```python
from build123d import *

# Parameters (mm, degrees)
F0_R      = 2.75
F1_DEPTH  = 4
F2_R      = 2.75
F3_DEPTH  = 9
F5_DEPTH  = 4
F7_R      = 5.125
F8_DEPTH  = 18.001
F10_DEPTH = 2


with BuildPart() as f1:
    # F0 (on Top) → F1 (new body)
    with BuildSketch(Plane.XY):
        with BuildLine():
            ThreePointArc((85, 25), (82.071068, 32.071068), (75, 35))
            Line((75, 35), (-75, 35))
            ThreePointArc((-75, 35), (-82.071068, 32.071068), (-85, 25))
            Line((-85, 25), (-85, -25))
            ThreePointArc((-85, -25), (-82.071068, -32.071068), (-75, -35))
            Line((-75, -35), (75, -35))
            ThreePointArc((75, -35), (82.071068, -32.071068), (85, -25))
            Line((85, -25), (85, 25))
        make_face()
        with Locations((-74, -25)):
            Circle(F0_R, mode=Mode.SUBTRACT)
        with Locations((74, -25)):
            Circle(F0_R, mode=Mode.SUBTRACT)
        with BuildLine():
            ThreePointArc((61.773717, 13.674819), (64.11513, 11.840019), (65, 9))
            Line((65, 9), (65, -9))
            ThreePointArc((65, -9), (64.11513, -11.840019), (61.773717, -13.674819))
            ThreePointArc((61.773717, -13.674819), (0, -25), (-61.773717, -13.674819))
            ThreePointArc((-61.773717, -13.674819), (-64.11513, -11.840019), (-65, -9))
            Line((-65, -9), (-65, 9))
            ThreePointArc((-65, 9), (-64.11513, 11.840019), (-61.773717, 13.674819))
            ThreePointArc((-61.773717, 13.674819), (0, 25), (61.773717, 13.674819))
        make_face(mode=Mode.SUBTRACT)
        with Locations((-74, 25)):
            Circle(F0_R, mode=Mode.SUBTRACT)
        with Locations((74, 25)):
            Circle(F0_R, mode=Mode.SUBTRACT)
    extrude(amount=F1_DEPTH)

    # F6: F3 across plane


with BuildPart() as f3:
    # F2 (on face) → F3 (new body)
    with BuildSketch(Plane(origin=(-85, 0, 0), x_dir=(0, -1, 0), z_dir=(-1, 0, 0))):
        with BuildLine():
            ThreePointArc((-17.318548, 7.163017), (-18.714839, 4.8897), (-21.23, 4))
            Line((-21.23, 4), (21.23, 4))
            ThreePointArc((21.23, 4), (18.714839, 4.8897), (17.318548, 7.163017))
            Line((17.318548, 7.163017), (15.676452, 14.836983))
            ThreePointArc((15.676452, 14.836983), (14.280161, 17.1103), (11.765, 18))
            Line((11.765, 18), (-11.765, 18))
            ThreePointArc((-11.765, 18), (-14.280161, 17.1103), (-15.676452, 14.836983))
            Line((-15.676452, 14.836983), (-17.318548, 7.163017))
        make_face()
        with Locations((-10.11, 11)):
            Circle(F2_R, mode=Mode.SUBTRACT)
        with Locations((10.11, 11)):
            Circle(F2_R, mode=Mode.SUBTRACT)
    extrude(amount=-F3_DEPTH)

    # F4 (on face) → F5 (cut)
    with BuildSketch(Plane.YZ.offset(-76)):
        Polygon((-5.202523, 11), (-7.656261, 15.25), (-12.563739, 15.25), (-15.017477, 11), (-12.563739, 6.75), (-7.656261, 6.75), align=None)
        Polygon((5.202523, 11), (7.656261, 6.75), (12.563739, 6.75), (15.017477, 11), (12.563739, 15.25), (7.656261, 15.25), align=None)
    extrude(amount=-F5_DEPTH, mode=Mode.SUBTRACT)


with BuildPart() as f1_1:
    add(f1.part)
    add(f3.part.mirror(Plane.YZ))


with BuildPart() as f8_tool:
    # F7 (on face) → F8 (new body, through all)
    with BuildSketch(Plane(origin=(0, 0, 0), x_dir=(1, 0, 0), z_dir=(0, 0, -1))):
        with Locations((-85, 0)):
            Circle(F7_R)
        with Locations((85, 0)):
            Circle(F7_R)
    extrude(amount=-F8_DEPTH)


with BuildPart() as f1_2:
    add(f1_1.part)

    # F8: cut by f8_tool
    add(f8_tool.part, mode=Mode.SUBTRACT)



with BuildPart() as f3_1:
    add(f3.part)

    # F8: cut by f8_tool
    add(f8_tool.part, mode=Mode.SUBTRACT)


with BuildPart() as f1_3:
    add(f1_2.part)

    add(f3_1.part)  # F10 merges F3
    # F9 (on Front) → F10 (join, symmetric)
    with BuildSketch(Plane.XZ):
        Polygon((-65, 4), (-76, 18), (-76, 4), align=None)
        Polygon((76, 4), (76, 18), (65, 4), align=None)
    extrude(amount=F10_DEPTH, both=True)


solid = f1_3.part
```
CAD build for the part. Positions are in the model's coordinates, mm. A direction names the side the tool comes from. Coordinates: 2 decimals unless noted, no trailing zeros. Order: outer loops, then holes, each group sorted by start corner. A loop starts at its lowest first (then second) coordinate and runs counter-clockwise, first axis right, second up.
(1) Saw through at D-D, the plane x = -2. Write the cut outline in (y, z), and give its area (3 significant figures).
Solution:
outline: (-35, 0) - (-24.99, 0) - (-24.99, 4) - (-35, 4) - close; (24.99, 0) - (35, 0) - (35, 4) - (24.99, 4) - close
area: 80.1 mm2
(2) Drill centre lines: L1, parallel to Y at x = -74, z = 2.6; L2, parallel to X at y = 7.5, z = 9.5; L3, parallel to Y at x = 75, z = 9. Where is each one in solid material? Low to high.
Solution:
L1: y = -35 to -27.75, -22.25 to 22.25, 27.75 to 35
L2: x = -85 to -80, 80 to 85
L3: y = -2 to 2
(3) Saw through at B-B, the plane x = 54. Write the cut outline in (y, z), and give its area (3 significant figures).
Solution:
outline: (-35, 0) - (-16.42, 0) - (-16.42, 4) - (-35, 4) - close; (16.42, 0) - (35, 0) - (35, 4) - (16.42, 4) - close
area: 149 mm2
(4) Saw through at C-C, the plane z = 2.5. Write the cut outline in (x, y) (3 decimals), and give its area (3 significant figures).
Solution:
outline: (-85, -25) arc R10 ccw to (-75, -35) - (75, -35) arc R10 ccw to (85, -25) - (85, -5.125) arc R5.125 cw to (85, 5.125) - (85, 25) arc R10 ccw to (75, 35) - (-75, 35) arc R10 ccw to (-85, 25) - (-85, 5.125) arc R5.125 cw to (-85, -5.125) - close; hole circle Ø5.5 at (-74, -25); hole circle Ø5.5 at (-74, 25); hole (-65, -9) arc R5 ccw to (-61.774, -13.675) arc R174.136 ccw to (61.774, -13.675) arc R5 ccw to (65, -9) - (65, 9) arc R5 ccw to (61.774, 13.675) arc R174.136 ccw to (-61.774, 13.675) arc R5 ccw to (-65, 9) - close; hole circle Ø5.5 at (74, -25); hole circle Ø5.5 at (74, 25)
area: 6,220 mm2
(5) Pin check, flat tips, straight feed: pin 1 Ø4.5 at (y, z) = (-1, 1) entering from -X; pin 2 Ø16.5 at (x, y) = (-4, -21) entering from +Z; pin 3 Ø4.5 at (y, z) = (-1.5, 2) entering from +X. Stop position of each tip, or through.
Solution:
pin 1: stops at x = -81.04
pin 2: stops at z = 4
pin 3: stops at x = 81.51
(6) Saw through at A-A, the plane y = 0. Write the cut outline in (x, z) (3 decimals), and give its area (4 significant figures).
Solution:
outline: (-79.875, 0) - (-65, 0) - (-65, 4) - (-76, 18) - (-79.875, 18) - close; (65, 0) - (79.875, 0) - (79.875, 18) - (76, 18) - (65, 4) - close
area: 381.5 mm2
(7) Mould opens along Z. For faces 5 (the face through (0.884, -24.998, 1.972)), 6 (the face through (80.6, 18.7, 4.9)), 7 (the face through (-77.972, 6.447, 13.155)) say: released by +Z, released by -Z, zero draft, split by the parting line, or undercut.
Solution:
face 5: zero draft
face 6: released by +Z
face 7: undercut
(8) Which spindle directions (+Z, -Z, +X, -X, +Y, -Y) get a long thin tool onto all of the face, cutting with end or side? Do faces 1 (the face through (-85, 13, 7)), 2 (the face through (-73, 2, 8)), 3 (the face through (77.972, 13.808, 13.095)), 4 (the face through (-73, -2, 8)). Say none if no direction does.
Solution:
face 1: +Z, -Z, -X, +Y, -Y
face 2: +Z, +Y
face 3: none
face 4: +Z, -Y
